Check sheet for the modelled part. Datum: model origin and axes. Units: mm. Give positions to 0.01 mm unless a question says otherwise; leave off trailing zeros. Write each loop counter-clockwise with the first axis right and the second up, starting at its lowest first coordinate (ties: lowest second). Pieces come first, ordered by that corner, then holes. Notation, with made-up numbers: (-18.75, -14) -> (-13.75, -14) arc R24 ccw to (-13.75, 8) -> close; hole circle Ø11 at (86.5, -31). An arc over 180 degrees is marked (long way). Use a Markdown table: item, result. Add a question column.
1. Gauge pin test, flat ends, axial feed: P1, Ø2, axis at x = -2.5, y = 1, coming from the +Z side; P2, Ø3, axis at x = 0, z = 0, coming from the -Y side. Record the tip position at first contact, or that the pin passes through.
2. Release check for a two-part mould opening along Z. For faces 1 (the cylindrical face through (-2.44, -0.03, -0.54)), 2 (the flat face through (1, -2, 3)), 3 (the flat face through (-2.025, -0.027, 3.45)) record: released by +Z, released by -Z, zero draft, split by the parting line, or undercut.
3. Scan lines: probe 1 along X at (y, z) = (1, 2); probe 2 along X at (y, z) = (-0.45, 0.75); probe 3 along Z at (x, y) = (-2, -1). Record each from-to range of solid material in increasing order. Write a range as [from, to].
4. Cross-section at A-A (z = 0). Enter the section's corners in (x, y) (3 decimals), then the cut area to 3 significant figures.
5. Cross-section at B-B (x = 0). Enter the section's corners in (y, z) (3 decimals).
6. Cross-section at C-C (y = 1.2). Enter the section's corners in (x, z), then the cut area to 3 significant figures.
from build123d import *

# Parameters (mm, degrees)
BOSS_EXTRUDE1_DEPTH      = 2
BOSS_EXTRUDE1_DEPTH_BACK = 2
SKETCH2_R                = 2.5
FILLET1_R                = 0.4
CUT_EXTRUDE2_DEPTH       = 0.15


with BuildPart() as part:
    # Sketch2 → Boss-Extrude1 (new, two sides: drawn at the far end of the back side and taken through both)
    with BuildSketch(Plane(origin=(0, 0, 0), x_dir=(1, 0, 0), z_dir=(0, 1, 0)).offset(-BOSS_EXTRUDE1_DEPTH_BACK)):
        Polygon((0, 4.618802154), (-4, 2.309401077), (-4, -2.309401077), (0, -4.618802154), (4, -2.309401077), (4, 2.309401077), align=None)
        with Locations(Location((0, 0, 0), (0, 0, 270))):
            Circle(SKETCH2_R, mode=Mode.SUBTRACT)
    extrude(amount=BOSS_EXTRUDE1_DEPTH + BOSS_EXTRUDE1_DEPTH_BACK)

    # Fillet1
    fillet1_edges = [part.edges().sort_by_distance(p)[0] for p in [
        (4, 0, -2.309401077),
        (4, 0, 2.309401077),
        (0, 0, 4.618802154),
        (-4, 0, 2.309401077),
        (-4, 0, -2.309401077),
        (0, 0, -4.618802154),
    ]]
    fillet(fillet1_edges, radius=FILLET1_R)

    # Sketch3 → Cut-Revolve2 (revolve, cut)
    with BuildSketch(Plane(origin=(0, 0, 0), x_dir=(0, 0, -1), z_dir=(1, 0, 0)), mode=Mode.PRIVATE) as cut_revolve2_sk:
        Polygon((3.9, -2), (4.618802154, -1.584999383), (4.618802154, -2), align=None)
        Polygon((2.5, 2), (2.5, 1.875), (2.625, 2), align=None)
        Polygon((2.5, -2), (2.5, -1.875), (2.625, -2), align=None)
        Polygon((3.9, 2), (4.618802154, 1.584999383), (4.618802154, 2), align=None)
    revolve(cut_revolve2_sk.sketch.rotate(Axis((0, -2, 0), (0, 1, 0)), 270), axis=Axis((0, -2, 0), (0, 1, 0)), mode=Mode.SUBTRACT)

    # Sketch12 → Cut-Extrude2 (cut)
    with BuildSketch(Plane(origin=(2, 0, 3.464101615), x_dir=(0.8660254037844384, 0, -0.5000000000000006), z_dir=(0.5000000000000006, 0, 0.8660254037844385))):
        Polygon((-0.747578096, 0), (-0.373789048, -0.647421623), (0.373789048, -0.647421623), (0.747578096, 0), (0.373789048, 0.647421623), (-0.373789048, 0.647421623), align=None)
    extrude(amount=-CUT_EXTRUDE2_DEPTH, mode=Mode.SUBTRACT)


solid = part.part
Worked answers:
| question | item | result |
|---|---|---|
| 1 | P1 | stops at z = 3.75 |
| 1 | P2 | passes through |
| 2 | face 1 | undercut |
| 2 | face 2 | zero draft |
| 2 | face 3 | released by +Z |
| 3 | probe 1 | x = [-4, -1.5], [1.5, 4] |
| 3 | probe 2 | x = [-4, -2.38], [2.38, 4] |
| 3 | probe 3 | z = [-3.46, -1.5], [1.5, 3.46] |
| 4 | outline | (-4, -1.942) -> (-3.9, -2) -> (-2.625, -2) -> (-2.5, -1.875) -> (-2.5, 1.875) -> (-2.625, 2) -> (-3.9, 2) -> (-4, 1.942) -> close; (2.5, -1.875) -> (2.625, -2) -> (3.9, -2) -> (4, -1.942) -> (4, 1.942) -> (3.9, 2) -> (2.625, 2) -> (2.5, 1.875) -> close |
| 4 | area | 12.0 mm² |
| 5 | outline | (-2, -3.9) -> (-1.621, -4.557) -> (1.621, -4.557) -> (2, -3.9) -> (2, -2.625) -> (1.875, -2.5) -> (-1.875, -2.5) -> (-2, -2.625) -> close; (-2, 2.625) -> (-1.875, 2.5) -> (1.875, 2.5) -> (2, 2.625) -> (2, 3.9) -> (1.621, 4.557) -> (-1.621, 4.557) -> (-2, 3.9) -> close |
| 6 | outline | (-4, -2.08) arc R0.4 ccw to (-3.8, -2.42) -> (-0.2, -4.5) arc R0.4 ccw to (0.2, -4.5) -> (3.8, -2.42) arc R0.4 ccw to (4, -2.08) -> (4, 2.08) arc R0.4 ccw to (3.8, 2.42) -> (0.2, 4.5) arc R0.4 ccw to (-0.2, 4.5) -> (-3.8, 2.42) arc R0.4 ccw to (-4, 2.08) -> close; hole circle Ø5 at (0, 0) |
| 6 | area | 35.7 mm² |
